```python
from build123d import *

# Parameters (mm, degrees)
SKETCH2_W               = 0.5
SKETCH2_H               = 0.5
BOSS_EXTRUDE1_DEPTH     = 2
CUT_EXTRUDE1_DEPTH      = 8.611008475
CUT_EXTRUDE1_DEPTH_BACK = 8.611008475
SKETCH3_W               = 3.125046629
SKETCH3_H               = 2.55575519


with BuildPart() as part:
    # Sketch1 → Revolve1 (revolve)
    with BuildSketch(Plane.XY, mode=Mode.PRIVATE) as revolve1_sk:
        with BuildLine():
            Line((0, -4.4), (0, 4.4))
            ThreePointArc((0, 4.4), (1.760695885, 3.670695885), (2.49, 1.91))
            Line((2.49, 1.91), (2.49, -3.669868996))
            Line((2.49, -3.669868996), (2.785, -3.669868996))
            Line((2.785, -3.669868996), (2.785, -4.4))
            Line((2.785, -4.4), (0, -4.4))
        make_face()
    revolve(revolve1_sk.sketch.rotate(Axis((0, -4.4, 0), (0, 1, 0)), 90), axis=Axis((0, -4.4, 0), (0, 1, 0)))

    # Sketch2 → Boss-Extrude1 (add)
    with BuildSketch(Plane.XZ.offset(4.4)):
        with Locations((0, -1.4)):
            Rectangle(SKETCH2_W, SKETCH2_H)
        with Locations((0, 1.4)):
            Rectangle(SKETCH2_W, SKETCH2_H)
    extrude(amount=BOSS_EXTRUDE1_DEPTH)

    # Sketch3 → Cut-Extrude1 (cut, two sides: drawn at the far end of the back side and taken through both)
    with BuildSketch(Plane(origin=(0.25, 0, 0), x_dir=(0, 0, -1), z_dir=(1, 0, 0)).offset(-CUT_EXTRUDE1_DEPTH_BACK)):
        with Locations((-1.351312101, -6.985445416)):
            Rectangle(SKETCH3_W, SKETCH3_H)
    extrude(amount=CUT_EXTRUDE1_DEPTH + CUT_EXTRUDE1_DEPTH_BACK, mode=Mode.SUBTRACT)


solid = part.part
```
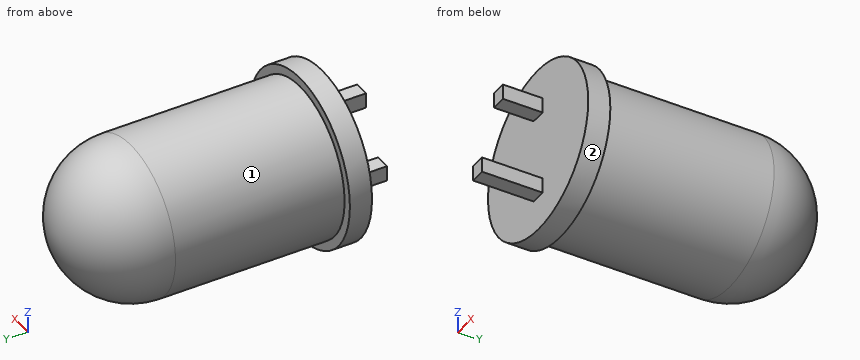
Here's how the part is built. I have some questions about the finished solid (model axes, mm). Face numbers are marked on the shaded views. A direction names the side the tool comes from. Round coordinates to 2 decimals unless told otherwise and drop trailing zeros. Order: outer loops, then holes, each group sorted by start corner. A loop starts at its lowest first (then second) coordinate and runs counter-clockwise, first axis right, second up. Notation, with made-up numbers: (82, 16) -> (102, 16) arc R15 ccw to (102, 31) -> close; hole circle Ø2 at (-19, -1.75). An arc over 180 degrees is marked (long way). Use a Markdown table: item, result. Add a question column.
(1) Suppose I cut it at A-A, the plane x = 0. Please give me the cut outline in (y, z) (3 decimals), and give its area (3 significant figures).
(2) For the marked faces 1 and 2, which set-ups out of +Z, -Z, +X, -X, +Y, -Y let a thin tool reach every point of the face, with its end or its side?
(3) I need wall thicknesses on line 1 along X through (y, z) = (1.25, -0.35); line 2 along X through (y, z) = (2.75, 0.75); line 3 along Y through (x, z) = (-1.6, -1.7). Which ranges of each line are inside material? Lowest first, please.
(4) For pin 1 Ø0.6 at (x, y) = (0, -5) entering from +Z; pin 2 Ø2 at (x, y) = (-1, 2.5) entering from -Z; pin 3 Ø1 at (x, y) = (-1, -1.5) entering from +Z, each with a flat end and sliding along its axis, tell me the tip position at first contact or that it passes through.
(5) Suppose I cut it at C-C, the plane y = -1.5. Please give me the cut outline in (x, z), and give its area (3 significant figures).
(6) Suppose I cut it at B-B, the plane z = 0. Please give me the cut outline in (x, y) (3 decimals).
(7) Suppose I cut it at D-D, the plane z = -2.2. Please give me the cut outline in (x, y).
Verdict:
| question | item | result |
|---|---|---|
| 1 | outline | (-6.4, -1.65) -> (-4.4, -1.65) -> (-4.4, -2.785) -> (-3.67, -2.785) -> (-3.67, -2.49) -> (1.91, -2.49) arc R2.49 ccw to (1.91, 2.49) -> (-3.67, 2.49) -> (-3.67, 2.785) -> (-4.4, 2.785) -> (-4.4, 1.65) -> (-5.708, 1.65) -> (-5.708, 1.15) -> (-4.4, 1.15) -> (-4.4, -1.15) -> (-6.4, -1.15) -> close |
| 1 | area | 43.2 mm2 |
| 2 | face 1 | +Y |
| 2 | face 2 | +Y, -Y |
| 3 | line 1 | -2.47 to 2.47 |
| 3 | line 2 | -2.22 to 2.22 |
| 3 | line 3 | -4.4 to 2.78 |
| 4 | pin 1 | z = 1.65 |
| 4 | pin 2 | z = -2.48 |
| 4 | pin 3 | z = 2.44 |
| 5 | outline | circle Ø4.98 at (0, 0) |
| 5 | area | 19.5 mm2 |
| 6 | outline | (-2.785, -4.4) -> (2.785, -4.4) -> (2.785, -3.67) -> (2.49, -3.67) -> (2.49, 1.91) arc R2.49 ccw to (-2.49, 1.91) -> (-2.49, -3.67) -> (-2.785, -3.67) -> close |
| 7 | outline | (-1.71, -4.4) -> (1.71, -4.4) -> (1.71, -3.67) -> (1.17, -3.67) -> (1.17, 1.91) arc R1.17 ccw to (-1.17, 1.91) -> (-1.17, -3.67) -> (-1.71, -3.67) -> close |
